```python
from build123d import *

# Parameters (mm, degrees)
F0_W     = 50.8
F0_H     = 38.1
F1_DEPTH = 31.75
F3_DEPTH = 50.801
F4_W     = 25.407727
F4_H     = 19.05
F5_DEPTH = 31.751


with BuildPart() as f1:
    # F0 (on Front) → F1 (new body)
    with BuildSketch(Plane.XZ):
        with Locations((25.4, 19.05)):
            Rectangle(F0_W, F0_H)
    extrude(amount=F1_DEPTH)

    # F2 (on face) → F3 (cut, through all)
    with BuildSketch(Plane.YZ.offset(50.8)):
        with BuildLine():
            Line((-31.75, 38.1), (-31.75, 12.7))
            ThreePointArc((-31.75, 12.7), (-13.78023, 20.13023), (-6.35, 38.1))
            Line((-6.35, 38.1), (-31.75, 38.1))
        make_face()
    extrude(amount=-F3_DEPTH, mode=Mode.SUBTRACT)

    # F4 (on face) → F5 (cut, through all)
    with BuildSketch(Plane(origin=(0, 0, 0), x_dir=(-1, 0, 0), z_dir=(0, 1, 0))):
        with Locations((-25.403863, 28.575)):
            Rectangle(F4_W, F4_H)
    extrude(amount=-F5_DEPTH, mode=Mode.SUBTRACT)


solid = f1.part
```
Geometry: final body of the model. Coordinates: model frame, mm. A direction names the side the tool comes from. Coordinates: 2 decimals unless noted, no trailing zeros. Order: outer loops, then holes, each group sorted by start corner. A loop starts at its lowest first (then second) coordinate and runs counter-clockwise, first axis right, second up. Notation, with made-up numbers: (26.5, -17) - (34.5, -17) arc R8 ccw to (34.5, -2) - close; hole circle Ø9 at (80, -39.75). An arc over 180 degrees is marked (long way). Write each question's results on one line, items separated by ' | '.
(1) Section query D-D, the plane x = 30. Return the cut outline in (y, z).
Values found:
outline: (-31.75, 0) - (0, 0) - (0, 19.05) - (-14.93, 19.05) arc R25.37 cw to (-31.75, 12.7) - close
(2) Section query A-A, the plane z = 27.5. Return the cut outline in (x, y).
Values found:
outline: (0, -8.66) - (12.7, -8.66) - (12.7, 0) - (0, 0) - close; (38.11, -8.66) - (50.8, -8.66) - (50.8, 0) - (38.11, 0) - close
(3) Section query C-C, the plane y = -3.5. Return the cut outline in (x, z).
Values found:
outline: (0, 0) - (50.8, 0) - (50.8, 38.1) - (38.11, 38.1) - (38.11, 19.05) - (12.7, 19.05) - (12.7, 38.1) - (0, 38.1) - close
(4) Section query B-B, the plane x = 42.5. Return the cut outline in (y, z).
Values found:
outline: (-31.75, 0) - (0, 0) - (0, 38.1) - (-6.35, 38.1) arc R25.37 cw to (-31.75, 12.7) - close
(5) First-contact query: pin 1 Ø12 at (x, y) = (21.5, -10.5) entering from +Z; pin 2 Ø1.5 at (x, z) = (9.5, 33) entering from -Y; pin 3 Ø10 at (x, y) = (39, -14.5) entering from +Z. Flat tips, straight axial feed; report the tip coordinate or a pass-through.
Values found:
pin 1: stops at z = 19.05 | pin 2: stops at y = -7.03 | pin 3: stops at z = 25.83
(6) Set-up query: faces 5 (the face through (25, -31.75, 6)), 6 (the face through (38.108, -4, 26)). Return all of +Z, -Z, +X, -X, +Y, -Y with unobstructed straight access to the full face (end or side cutting, diameter ignored); none if empty.
Values found:
face 5: +Z, -Z, +X, -X, -Y | face 6: +Z, +Y, -Y
(7) Mould query, pull axis X, two halves, no side actions, for faces 1 (the face through (12.7, -4, 26)), 2 (the face through (26, -7, 19.05)), 3 (the face through (50.8, -12, 15)), 4 (the face through (44, -3, 38.1)). Classes: +X half, -X half, draft (parallel to the pull), parting line (faces both ways), or undercut.
Values found:
face 1: undercut | face 2: undercut | face 3: +X half | face 4: draft
(8) Line query: line 1 (X direction, y = -5, z = 30.5); line 2 (Z direction, x = 30, y = -13); line 3 (Z direction, x = 16.5, y = -29.5). Output: solid intervals per line, ascending. Write a range as [from, to].
Values found:
line 1: x = [0, 12.7], [38.11, 50.8] | line 2: z = [0, 19.05] | line 3: z = [0, 12.8]
